Job drawing, mm, ordinate dimensions from the low corner. One solid piece. Give positions to 0.01 mm unless a question says otherwise; leave off trailing zeros. Loops run counter-clockwise (first coordinate to the right, second up) from the corner with the lowest first, then second, coordinate; pieces in that order, holes last. Notation, with made-up numbers: (59, 32.5) -> (92, 32.5) arc R16 ccw to (92, 59.5) -> close; hole circle Ø11 at (25, 28.25). An arc over 180 degrees is marked (long way). Use one line per item in the form item = value.
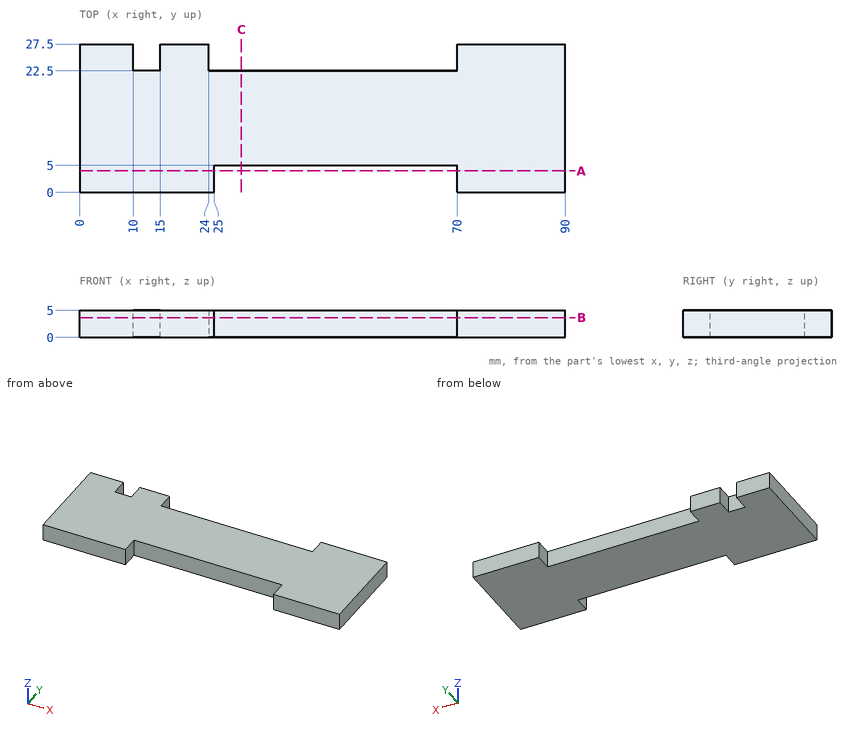
1. Drop flat-ended pins along their axis: P1, Ø2.5, axis at x = 13, z = 3, coming from the +Y side; P2, Ø3, axis at x = 50.5, z = 2, coming from the -Y side. Give the stop position or say it passes through.
Result sheet:
P1 = 22.5
P2 = 5
2. Cut at B-B, the plane z = 3.65. Write the cut outline in (x, y).
Result sheet:
outline = (0, 0) -> (25, 0) -> (25, 5) -> (70, 5) -> (70, 0) -> (90, 0) -> (90, 27.5) -> (70, 27.5) -> (70, 22.5) -> (24, 22.5) -> (24, 27.5) -> (15, 27.5) -> (15, 22.5) -> (10, 22.5) -> (10, 27.5) -> (0, 27.5) -> close
3. Cut at C-C, the plane x = 30. Write the cut outline in (y, z), then the cut area to 3 significant figures.
Result sheet:
outline = (5, 0) -> (22.5, 0) -> (22.5, 5) -> (5, 5) -> close
area = 87.5 mm^2
4. Cut at A-A, the plane y = 4. Write the cut outline in (x, z), then the cut area to 3 significant figures.
Result sheet:
outline = (0, 0) -> (25, 0) -> (25, 5) -> (0, 5) -> close; (70, 0) -> (90, 0) -> (90, 5) -> (70, 5) -> close
area = 225 mm^2
5. Drill centre lines: line 1 (X direction, y = 1.5, z = 0.7); line 2 (Y direction, x = 12, z = 2.35); line 3 (Y direction, x = 49, z = 3.8). Where is each one in solid material? Low to high.
Result sheet:
line_1 = 0 to 25, 70 to 90
line_2 = 0 to 22.5
line_3 = 5 to 22.5
